For this review, use the dimensioned drawing (mm, ordinates from the lowest corner) and the shaded views. Coordinates: 2 decimals unless noted, no trailing zeros. Loops run counter-clockwise (first coordinate to the right, second up) from the corner with the lowest first, then second, coordinate; pieces in that order, holes last.
1. Take a section at A-A, the plane x = 3. State the section outline as (y, z) points.
2. Clearance check with flat-ended pins moving along their axes: P1, Ø2, axis at x = 1, z = 5, coming from the -Y side; P2, Ø1.3, axis at x = 3, y = 19, coming from the -Z side; P3, Ø0.6, axis at x = 3, z = 3, coming from the +Y side. State where each tip first meets the part, or that it passes through.
3. Mouldability with a two-part tool opening along X and no side actions: class the marked faces 1, 2, 3 and 4 as pulls with the +X half, pulls with the -X half, needs draft (parallel to the pull), parting line crosses it, or undercut.
4. Take a section at B-B, the plane y = 7. State the section outline as (x, z) points.
5. To check wall thickness, follow probe 1 along X at (y, z) = (5.25, 3.1); probe 2 along Y at (x, z) = (3, 2.9); probe 3 along Z at (x, y) = (2.75, 10.5). State the ranges of each line that lie inside material, in increasing order.
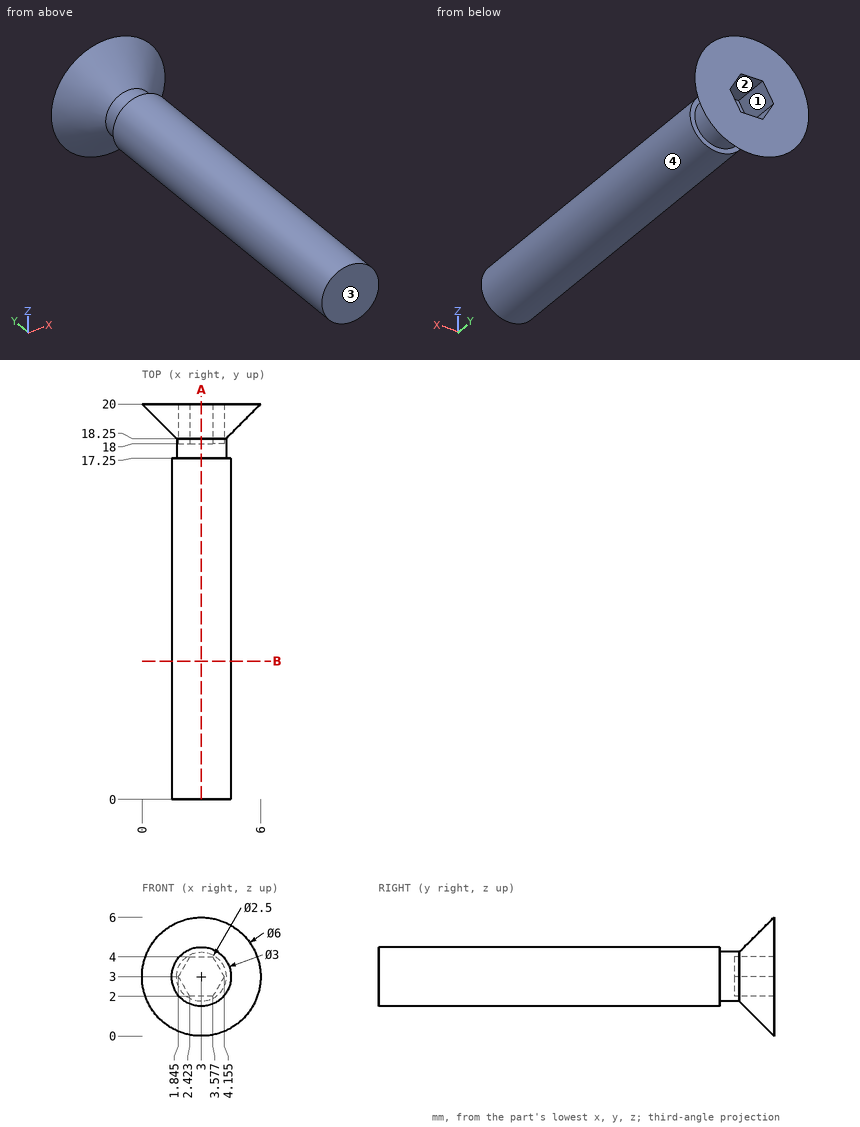
Results list:
1. outline: (0, 1.5) - (17.25, 1.5) - (17.25, 1.75) - (18.25, 1.75) - (20, 0) - (20, 2) - (18, 2) - (18, 4) - (20, 4) - (20, 6) - (18.25, 4.25) - (17.25, 4.25) - (17.25, 4.5) - (0, 4.5) - close
2. P1: stops at y = 18.83
2. P2: stops at z = 0.35
2. P3: stops at y = 18
3. face 1: undercut
3. face 2: undercut
3. face 3: needs draft
3. face 4: parting line crosses it
4. outline: circle Ø3 at (3, 3)
5. probe 1: x = 1.5 to 4.5
5. probe 2: y = 0 to 18
5. probe 3: z = 1.52 to 4.48
